Autodesk Inventor part; units mm, degrees
ref_plane "YZ Plane" through (0, 0, 0) normal (1, 0, 0) x (0, 1, 0)
ref_plane "XZ Plane" through (0, 0, 0) normal (0, 1, 0) x (-1, 0, 0)
ref_plane "XY Plane" through (0, 0, 0) normal (0, 0, 1) x (1, 0, 0)
sketch "Sketch1" plane through (0, 0, 0) normal (0, 1, 0) x (-1, 0, 0)
  line L0 (-10, 10) -> (10, 10)
  line L1 (10, 10) -> (10, -10)
  line L2 (10, -10) -> (-10, -10)
  line L3 (-10, -10) -> (-10, 10)
  point P0 (0, 0)
  dimension "d0" = 20
  dimension "d1" = 20
  dimension "d2" = 10
  dimension "d3" = 10
extrude "Extrusion1" add sketch "Sketch1" along normal blind 20
sketch "Sketch2" plane through (0, 0, 0) normal (0, -1, 0) x (1, 0, 0)
  line L0 (15, -15) -> (-35, -15)
  line L1 (-35, -15) -> (-35, 15)
  line L2 (-35, 15) -> (-15, 35)
  line L3 (-15, 35) -> (15, 35)
  line L4 (15, 35) -> (15, -15)
  line L5 (10, -10) -> (-10, -10)
  line L6 (10, 10) -> (10, -10)
  point P0 (0, 0)
  dimension "d6" = 5
  dimension "d7" = 5
  dimension "d8" = 135
  dimension "d9" = 30
  dimension "d10" = 30
  dimension "d11" = 50
extrude "Extrusion2" add sketch "Sketch2" along normal blind 5
sketch "Sketch4" plane through (0, 0, 0) normal (0, 1, 0) x (1, 0, 0)
  point P0 (0, 0)
sketch "Sketch5" plane through (0, 0, 0) normal (0, 1, 0) x (1, 0, 0)
  point P0 (0, 0)
sketch "Sketch6" plane through (0, 0, 0) normal (0, 1, 0) x (1, 0, 0)
  line L0 (10, -30) -> (10, 10)
  line L1 (10, 10) -> (-30, 10)
  line L2 (-30, 10) -> (-30, 15)
  line L3 (-30, 15) -> (15, 15)
  line L4 (15, 15) -> (15, -30)
  line L5 (15, -30) -> (10, -30)
  line L6 (15, -35) -> (-15, -35)
  line L7 (-35, -15) -> (-35, 15)
  point P0 (0, 0)
  dimension "d18" = 5
  dimension "d21" = 5
extrude "Extrusion4" add sketch "Sketch6" along normal blind 20
sketch "Sketch7" plane through (0, 20, 0) normal (0, 1, 0) x (1, 0, 0)
  line L0 (-10, 10) -> (-30, 10)
  line L1 (-30, 10) -> (-30, 15)
  line L2 (-35, 15) -> (-30, 15)
  line L3 (-35, -15) -> (-35, 15)
  line L4 (-15, -35) -> (-35, -15)
  line L5 (15, -35) -> (-15, -35)
  line L6 (15, -30) -> (15, -35)
  line L7 (15, -30) -> (10, -30)
  line L8 (10, -30) -> (10, -10)
  line L9 (-10, -10) -> (10, -10)
  line L10 (-10, 10) -> (-10, -10)
  line L11 (-10, 10) -> (-10, -10)
  line L12 (-10, -10) -> (10, -10)
  line L13 (10, -10) -> (10, -30)
  line L14 (10, -30) -> (15, -30)
  line L15 (15, -30) -> (15, 15)
  line L16 (15, 15) -> (-30, 15)
  line L17 (-30, 15) -> (-30, 10)
  line L18 (-30, 10) -> (-10, 10)
  line L19 (15, -35) -> (-15, -35)
  line L20 (-15, -35) -> (-35, -15)
  line L21 (-35, -15) -> (-35, 15)
  line L22 (-35, 15) -> (15, 15)
  line L23 (15, 15) -> (15, -35)
  point P0 (0, 0)
extrude "Extrusion5" add sketch "Sketch7" along normal blind 5
sketch "Sketch8" plane through (10, 0, 30) normal (0, 0, 1) x (1, 0, 0)
  line L0 (5, 20) -> (0, 20)
  line L1 (0, 20) -> (0, 0)
  line L2 (0, 0) -> (5, 0)
  line L3 (5, 0) -> (5, 20)
  point P0 (-10, 0)
extrude "Extrusion6" add sketch "Sketch8" along normal blind 5
sketch "Sketch9" plane through (-30, 0, -15) normal (-1, 0, 0) x (0, 0, 1)
  line L0 (5, 20) -> (0, 20)
  line L1 (0, 20) -> (0, 0)
  line L2 (0, 0) -> (5, 0)
  line L3 (5, 0) -> (5, 20)
  point P0 (15, 0)
extrude "Extrusion7" add sketch "Sketch9" along normal blind 5
sketch "Sketch13" plane through (15, -5, -15) normal (0, 0, -1) x (-1, 0, 0)
  line L0 (25, 5) -> (25, 25)
  line L1 (50, 25) -> (25, 25)
  line L2 (50, 5) -> (50, 25)
  line L3 (25, 5) -> (50, 5)
  line L4 (37.5, 5) -> (50, 5) construction
  line L5 (50, 5) -> (50, 15) construction
  line L6 (50, 15) -> (37.5, 15) construction
  line L7 (37.5, 15) -> (37.5, 5) construction
  point P0 (15, 5)
  dimension "d32" = 12.5
  dimension "d33" = 10
sketch "Sketch14" plane through (15, -5, 35) normal (1, 0, 0) x (0, 0, -1)
  line L0 (25, 5) -> (25, 25)
  line L1 (0, 5) -> (25, 5)
  line L2 (0, 25) -> (0, 5)
  line L3 (25, 25) -> (0, 25)
  line L4 (12.5, 15) -> (0, 15) construction
  line L5 (0, 15) -> (0, 25) construction
  line L6 (0, 25) -> (12.5, 25) construction
  line L7 (12.5, 25) -> (12.5, 15) construction
  point P0 (35, 5)
  dimension "d34" = 12.5
  dimension "d35" = 10
hole "Hole1" at (15, 10, 22.5) direction (-1, 0, 0) diameter 3.4 end through all counterbore diameter 6.5 counterbore depth 3
hole "Hole2" at (-22.5, 10, -15) direction (0, 0, 1) diameter 3.4 end through all counterbore diameter 6.5 counterbore depth 3
fillet "Fillet1" radius 10 1 edges at (15, 10, -15)
fillet "Fillet2" radius 5 6 edges at (12.0711, -5, -12.0711) (15, -5, 15) (-15, -5, -15) (12.0711, 25, -12.0711) (15, 25, 15) (-15, 25, -15)
fillet "Fillet3" radius 2 12 edges at (-25, 25, 25) (13.5355, 23.5355, 35) (15, 10, 35) (13.5355, -3.5355, 35) (-2.5, -5, 35) (-2.5, 25, 35) (-25, -5, 25) (-35, -3.5355, -13.5355) (-35, 10, -15) (-35, 23.5355, -13.5355) (-35, 25, 2.5) (-35, -5, 2.5)
properties part number "flat_corner" material "ABS Plastic"
Verification items for the finished model (mm, model axes). A direction names the side the tool comes from. Give positions to 0.01 mm unless a question says otherwise; leave off trailing zeros. Order: outer loops, then holes, each group sorted by start corner. A loop starts at its lowest first (then second) coordinate and runs counter-clockwise, first axis right, second up. Notation, with made-up numbers: M 48.5,24 L 105.5,24 A22 cw 105.5,63 Z; hole C 17,30.25 d6. An arc over 180 degrees is marked long. Return JSON: item names as keys, results as strings. Group by question number.
1) Access from +Z, -Z, +X, -X, +Y, -Y to the whole of each face (thin tool, end or side, straight path). Record for faces 5 (the face through (-2.33, 24.43, 34.4)), 6 (the face through (-13, 0, 13)), 7 (the face through (12, 11.4, 21.1)).
2) Scan lines: line 1 (Y direction, x = -25, z = 3.5); line 2 (Z direction, x = -8.5, y = 8.5); line 3 (Z direction, x = -16, y = 12.25). Record each from-to range of solid material in increasing order.
3) Section check C-C on y = 14.5. Record the cut outline in (x, z).
4) Section check A-A on y = 10. Record the cut outline in (x, z), and give its area (3 significant figures).
5) Mould release check, pull along Y, two halves, no side actions. Record for faces 1 (the face through (-35, 10.1, -10.5)), 2 (the face through (-34.43, -4.4, 2.68)), 3 (the face through (-20.522, 7.421, -13.479)), 4 (the face through (-14, 23, -14)): pulls with the +Y half, pulls with the -Y half, needs draft (parallel to the pull), parting line crosses it, or undercut.
6) Section check B-B on z = 6. Record the cut outline in (x, y).
7) Go/stop test with flat-tipped pins: pin 1 Ø10.5 at (y, z) = (10, 22.5) entering from -X; pin 2 Ø6 at (x, y) = (-21, 15.5) entering from +Z; pin 3 Ø12 at (x, y) = (-5, 8.5) entering from +Z; pin 4 Ø2.5 at (y, z) = (10, 22.5) entering from +X. Record where each tip stops, or that it passes through.
Answer block:
{
 "1": {"face 5": "+Z, +X, -X, +Y", "face 6": "+Z, -X", "face 7": "+X"},
 "2": {"line 1": "y = -5 to 0, 20 to 25", "line 2": "z = -15 to 10", "line 3": "z = -15 to -10"},
 "3": {"outline": "M -35,-13 A2 ccw -33,-15 L 5,-15 A10 ccw 15,-5 L 15,33 A2 ccw 13,35 L 10,35 L 10,10 L -10,10 L -10,-10 L -35,-10 Z"},
 "4": {"outline": "M -35,-13 A2 ccw -33,-15 L -25.75,-15 L -25.75,-12 L -24.2,-12 L -24.2,-10 L -35,-10 Z; M -20.8,-12 L -19.25,-12 L -19.25,-15 L 5,-15 A10 ccw 15,-5 L 15,19.25 L 12,19.25 L 12,20.8 L 10,20.8 L 10,10 L -10,10 L -10,-10 L -20.8,-10 Z; M 10,24.2 L 12,24.2 L 12,25.75 L 15,25.75 L 15,33 A2 ccw 13,35 L 10,35 Z", "area": "799 mm^2"},
 "5": {"face 1": "needs draft", "face 2": "pulls with the -Y half", "face 3": "undercut", "face 4": "pulls with the +Y half"},
 "6": {"outline": "M -35,-3 A2 ccw -33,-5 L 10,-5 A5 ccw 15,0 L 15,20 A5 ccw 10,25 L -33,25 A2 ccw -35,23 L -35,20 L -10,20 L -10,0 L -35,0 Z"},
 "7": {"pin 1": "stops at x = 10", "pin 2": "stops at z = -10", "pin 3": "stops at z = 10", "pin 4": "passes through"}
}
